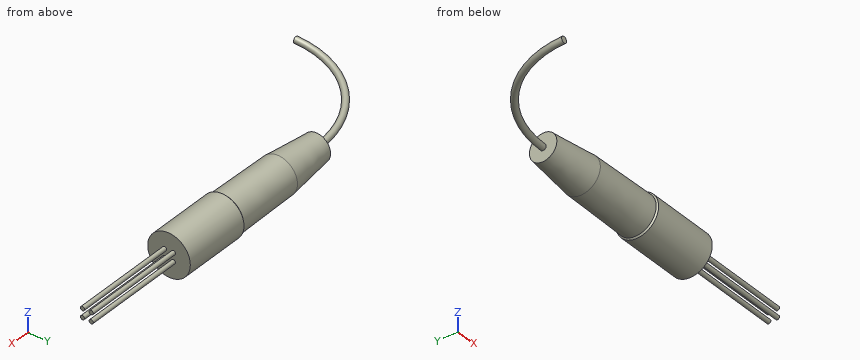
from build123d import *

# Parameters (mm, degrees)
CHAMFER_1_SIZE  = 0.2
SKETCH_4_R      = 0.45
SKETCH_5_R      = 0.3
EXTRUDE_2_DEPTH = 15


with BuildPart() as part:
    # 旋转2: read off the stored shape, not the designer's step
    # 旋转2 outline → 旋转2 (revolve)
    with BuildSketch(Plane.YX):
        Polygon((3.1, 0), (0, 0), (0, -27), (2, -27), (2.75, -20), (2.9, -10), (3.1, -10), align=None)
    revolve(axis=Axis((0, 0, 0), (1, 0, 0)))

    # 倒角1
    chamfer_1_edges = [part.edges().sort_by_distance(p)[0] for p in [
        (-10, -3.1, 0),
    ]]
    chamfer(chamfer_1_edges, length=CHAMFER_1_SIZE - 0.0001)  # a hair under: the kernel refuses the full size

    # 扫描1: sweep along a path in 草图3
    with BuildLine(Plane.XY) as sweep_1_path:
        ThreePointArc((-27, 0), (-37.606601718, -4.393398282), (-42, -15))
    # 草图4 → 扫描1 (sweep)
    with BuildSketch(Plane.ZY.offset(27)):
        Circle(SKETCH_4_R)
    sweep(path=sweep_1_path.line)

    # 草图5 → 拉伸2 (add)
    with BuildSketch(Plane(origin=(0, 0, 0), x_dir=(0, 0, -1), z_dir=(1, 0, 0))):
        with Locations(Location((-0.635, 0.635, 0), (0, 0, 270))):
            Circle(SKETCH_5_R)
        with Locations(Location((-0.635, -0.635, 0), (0, 0, 270))):
            Circle(SKETCH_5_R)
        with Locations(Location((0.635, 0.635, 0), (0, 0, 270))):
            Circle(SKETCH_5_R)
        with Locations(Location((0.635, -0.635, 0), (0, 0, 270))):
            Circle(SKETCH_5_R)
    extrude(amount=EXTRUDE_2_DEPTH)


solid = part.part
Verification items for the finished model (mm, model axes). Coordinates: 2 decimals unless noted, no trailing zeros. Write each loop counter-clockwise with the first axis right and the second up, starting at its lowest first coordinate (ties: lowest second). Pieces come first, ordered by that corner, then holes. Notation, with made-up numbers: (-8, 21.5) -> (8, 21.5) arc R21 ccw to (8, 40.5) -> close; hole circle Ø3 at (24, 67.25). An arc over 180 degrees is marked (long way). One line per item, written item: value. Start each with the question number.
Q1. Go/stop test with flat-tipped pins: P1, Ø2, axis at y = -9.5, z = 0, coming from the -X side; P2, Ø3, axis at x = -33.5, z = 1.5, coming from the +Y side; P3, Ø3, axis at y = -12.5, z = -2, coming from the -X side; P4, Ø1.5, axis at y = -7, z = -1, coming from the +X side. Record where each tip stops, or that it passes through.
Q2. Cross-section at B-B on x = 5.5. Enter the section's corners in (y, z) (3 decimals).
Q3. Cross-section at A-A on x = -9. Enter the section's corners in (y, z).
Q4. Thickness scan on L1, parallel to X at y = -1.75, z = -0.5; L2, parallel to Y at x = -24, z = 1 (3 decimals); L3, parallel to Z at x = -13, y = 0.5. Record the ranges inside material, lowest first. Write a range as from..to.
Checked values:
1. P1: stops at x = -41.78
1. P2: stops at y = -0.71
1. P3: passes through
1. P4: stops at x = -39.1
2. outline: circle Ø0.6 at (-0.635, -0.635); circle Ø0.6 at (-0.635, 0.635); circle Ø0.6 at (0.635, -0.635); circle Ø0.6 at (0.635, 0.635)
3. outline: circle Ø6.2 at (0, 0)
4. L1: x = -27..0
4. L2: y = -2.095..2.095
4. L3: z = -2.81..2.81
